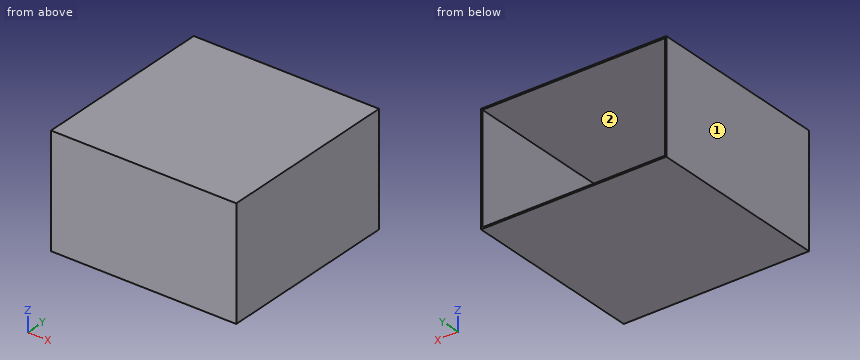
```python
from build123d import *

# Parameters (mm, degrees)
SKETCH_1_W          = 250
SKETCH_1_H          = 250
EXTRUDE_2_DEPTH     = 150
CUT_EXTRUDE_START   = 250
SKETCH_3_W          = 246
SKETCH_3_H          = 146
CUT_EXTRUDE_1_DEPTH = 248


with BuildPart() as part:
    # 草图1 → 凸台-拉伸2 (new body)
    with BuildSketch(Plane.XY):
        with Locations((125, 125)):
            Rectangle(SKETCH_1_W, SKETCH_1_H)
    extrude(amount=EXTRUDE_2_DEPTH)

    # 草图3 → 切除-拉伸1 (cut)
    with BuildSketch(Plane(origin=(0, 0, 0), x_dir=(1, 0, 0), z_dir=(0, 1, 0)).offset(CUT_EXTRUDE_START)):
        with Locations((125, -75)):
            Rectangle(SKETCH_3_W, SKETCH_3_H)
    extrude(amount=-CUT_EXTRUDE_1_DEPTH, mode=Mode.SUBTRACT)


solid = part.part
```
Model file for the job. Use its own axes, mm. Face numbers are marked on the shaded views. A direction names the side the tool comes from. Coordinates: 2 decimals unless noted, no trailing zeros. Loops run counter-clockwise (first coordinate to the right, second up) from the corner with the lowest first, then second, coordinate; pieces in that order, holes last. Notation, with made-up numbers: (-33.5, -17) - (-27.5, -17) arc R29 ccw to (-27.5, 13) - close; hole circle Ø8 at (-31, -18). An arc over 180 degrees is marked (long way). Write item = value, one per line. Start each with the question number.
Item 1: Saw through at C-C, the plane z = 81.5. List the corners of the cut face in (x, y).
Item 2: Drop flat-ended pins along their axis: pin 1 Ø1.5 at (y, z) = (33, 44) entering from -X; pin 2 Ø6 at (x, z) = (39, 80) entering from +Y. Give the stop position or say it passes through.
Item 3: Saw through at B-B, the plane x = 154. List the corners of the cut face in (y, z).
Item 4: 3-axis set-ups, long thin cutter, end or side, ignore diameter. For the marked faces 1 and 2: which of +Z, -Z, +X, -X, +Y, -Y reach the whole face in a straight line?
Item 5: Wall check: probe 1 along X at (y, z) = (26.5, 35); probe 2 along Z at (x, y) = (209, 23.5); probe 3 along Y at (x, z) = (97, 60). Give the ranges that are in metal, low to high. Write a range as [from, to].
Item 6: Saw through at A-A, the plane y = 112. List the corners of the cut face in (x, z), then the cut area to 3 significant figures.
Answers:
q1.outline = (0, 0) - (250, 0) - (250, 250) - (248, 250) - (248, 2) - (2, 2) - (2, 250) - (0, 250) - close
q2.pin_1 = 0
q2.pin_2 = 2
q3.outline = (0, 0) - (250, 0) - (250, 2) - (2, 2) - (2, 148) - (250, 148) - (250, 150) - (0, 150) - close
q4.face_1 = +Z, -Z, -X, +Y, -Y
q4.face_2 = +Y
q5.probe_1 = [0, 2], [248, 250]
q5.probe_2 = [0, 2], [148, 150]
q5.probe_3 = [0, 2]
q6.outline = (0, 0) - (250, 0) - (250, 150) - (0, 150) - close; hole (2, 2) - (248, 2) - (248, 148) - (2, 148) - close
q6.area = 1,580 mm2
